from build123d import *

# Parameters (mm, degrees)
F0_R          = 3
F0_R_2        = 2.5
F1_DEPTH      = 408.599
F2_R          = 2
F3_R          = 7
F5_DEPTH      = 30
F5_DEPTH_BACK = 30


# Not quite as in the source:
# - a feature names something its author has since deleted; it is built from what else it names


with BuildPart() as f1:
    # F0 (on Top) → F1 (new body)
    with BuildSketch(Plane.XY):
        with BuildLine():
            Line((18.15, -30), (30, -30))
            Line((30, -30), (30, -18.15))
            Line((30, -18.15), (27.5, -18.15))
            Line((27.5, -18.15), (27.5, -20.15))
            Line((27.5, -20.15), (21.5477069044, -20.15))
            ThreePointArc((21.5477069044, -20.15), (19.5, -15), (21.5477069044, -9.85))
            Line((21.5477069044, -9.85), (27.5, -9.85))
            Line((27.5, -9.85), (27.5, -11.85))
            Line((27.5, -11.85), (30, -11.85))
            Line((30, -11.85), (30, 11.85))
            Line((30, 11.85), (27.5, 11.85))
            Line((27.5, 11.85), (27.5, 9.85))
            Line((27.5, 9.85), (21.5477069044, 9.85))
            ThreePointArc((21.5477069044, 9.85), (19.5, 15), (21.5477069044, 20.15))
            Line((21.5477069044, 20.15), (27.5, 20.15))
            Line((27.5, 20.15), (27.5, 18.15))
            Line((27.5, 18.15), (30, 18.15))
            Line((30, 18.15), (30, 30))
            Line((30, 30), (18.15, 30))
            Line((18.15, 30), (18.15, 27.5))
            Line((18.15, 27.5), (20.15, 27.5))
            Line((20.15, 27.5), (20.15, 21.5477069044))
            ThreePointArc((20.15, 21.5477069044), (15, 19.5), (9.85, 21.5477069044))
            Line((9.85, 21.5477069044), (9.85, 27.5))
            Line((9.85, 27.5), (11.85, 27.5))
            Line((11.85, 27.5), (11.85, 30))
            Line((11.85, 30), (-11.85, 30))
            Line((-11.85, 30), (-11.85, 27.5))
            Line((-11.85, 27.5), (-9.85, 27.5))
            Line((-9.85, 27.5), (-9.85, 21.5477069044))
            ThreePointArc((-9.85, 21.5477069044), (-15, 19.5), (-20.15, 21.5477069044))
            Line((-20.15, 21.5477069044), (-20.15, 27.5))
            Line((-20.15, 27.5), (-18.15, 27.5))
            Line((-18.15, 27.5), (-18.15, 30))
            Line((-18.15, 30), (-30, 30))
            Line((-30, 30), (-30, 18.15))
            Line((-30, 18.15), (-27.5, 18.15))
            Line((-27.5, 18.15), (-27.5, 20.15))
            Line((-27.5, 20.15), (-21.5477069044, 20.15))
            ThreePointArc((-21.5477069044, 20.15), (-19.5, 15), (-21.5477069044, 9.85))
            Line((-21.5477069044, 9.85), (-27.5, 9.85))
            Line((-27.5, 9.85), (-27.5, 11.85))
            Line((-27.5, 11.85), (-30, 11.85))
            Line((-30, 11.85), (-30, -11.85))
            Line((-30, -11.85), (-27.5, -11.85))
            Line((-27.5, -11.85), (-27.5, -9.85))
            Line((-27.5, -9.85), (-21.5477069044, -9.85))
            ThreePointArc((-21.5477069044, -9.85), (-19.5, -15), (-21.5477069044, -20.15))
            Line((-21.5477069044, -20.15), (-27.5, -20.15))
            Line((-27.5, -20.15), (-27.5, -18.15))
            Line((-27.5, -18.15), (-30, -18.15))
            Line((-30, -18.15), (-30, -30))
            Line((-30, -30), (-18.15, -30))
            Line((-18.15, -30), (-18.15, -27.5))
            Line((-18.15, -27.5), (-20.15, -27.5))
            Line((-20.15, -27.5), (-20.15, -21.5477069044))
            ThreePointArc((-20.15, -21.5477069044), (-15, -19.5), (-9.85, -21.5477069044))
            Line((-9.85, -21.5477069044), (-9.85, -27.5))
            Line((-9.85, -27.5), (-11.85, -27.5))
            Line((-11.85, -27.5), (-11.85, -30))
            Line((-11.85, -30), (11.85, -30))
            Line((11.85, -30), (11.85, -27.5))
            Line((11.85, -27.5), (9.85, -27.5))
            Line((9.85, -27.5), (9.85, -21.5477069044))
            ThreePointArc((9.85, -21.5477069044), (15, -19.5), (20.15, -21.5477069044))
            Line((20.15, -21.5477069044), (20.15, -27.5))
            Line((20.15, -27.5), (18.15, -27.5))
            Line((18.15, -27.5), (18.15, -30))
        make_face()
        with Locations((-25, -25)):
            Circle(F0_R, mode=Mode.SUBTRACT)
        with Locations((-15, -15)):
            Circle(F0_R_2, mode=Mode.SUBTRACT)
        with Locations((25, -25)):
            Circle(F0_R, mode=Mode.SUBTRACT)
        with Locations((15, -15)):
            Circle(F0_R_2, mode=Mode.SUBTRACT)
        with Locations((-25, 25)):
            Circle(F0_R, mode=Mode.SUBTRACT)
        with Locations((-15, 15)):
            Circle(F0_R_2, mode=Mode.SUBTRACT)
        Polygon((-7, 22), (-7, 27.5), (0, 27.5), (7, 27.5), (7, 22), (10, 16), (10, 10), (16, 10), (22, 7), (27.5, 7), (27.5, 0), (27.5, -7), (22, -7), (16, -10), (10, -10), (10, -16), (7, -22), (7, -27.5), (0, -27.5), (-7, -27.5), (-7, -22), (-10, -16), (-10, -10), (-16, -10), (-22, -7), (-27.5, -7), (-27.5, 0), (-27.5, 7), (-22, 7), (-16, 10), (-10, 10), (-10, 16), align=None, mode=Mode.SUBTRACT)
        with Locations((15, 15)):
            Circle(F0_R_2, mode=Mode.SUBTRACT)
        with Locations((25, 25)):
            Circle(F0_R, mode=Mode.SUBTRACT)
    extrude(amount=F1_DEPTH)

    # F2
    f2_edges = [f1.edges().sort_by_distance(p)[0] for p in [
        (-7, 27.5, 204.2995),
        (7, 27.5, 204.2995),
    ]]
    fillet(f2_edges, radius=F2_R)

    # F3
    f3_edges = [f1.edges().sort_by_distance(p)[0] for p in [
        (-10, 16, 204.2995),
        (10, 16, 204.2995),
    ]]
    fillet(f3_edges, radius=F3_R)

    # F4 (on Right) → F5 (cut, two sides)
    with BuildSketch(Plane.YZ) as f5_sk:
        Polygon((-164.2855995683, 38.6458085579), (-188.5911429791, -83.5464097089), (5.6944565892, -122.1922182668), (30, 0), align=None)
    extrude(amount=F5_DEPTH, mode=Mode.SUBTRACT)
    extrude(f5_sk.sketch, amount=-F5_DEPTH_BACK, mode=Mode.SUBTRACT)


solid = f1.part
Read the model definition and answer for the solid it produces. Units are mm, in the model's axes. A direction names the side the tool comes from. Give positions to 0.01 mm unless a question says otherwise; leave off trailing zeros. Write each loop counter-clockwise with the first axis right and the second up, starting at its lowest first coordinate (ties: lowest second). Pieces come first, ordered by that corner, then holes. Notation, with made-up numbers: (2, -27) -> (59, -27) arc R16 cw to (59, -14) -> close; hole circle Ø2 at (-39, 53). An arc over 180 degrees is marked (long way). Answer as a JSON object with one key per item and string values. Group by question number.
1) The mould has two halves that part along Y. Classify faces 3 (the flat face through (27.5, 0, 204)), 4 (the flat face through (0, 30, 201)), 5 (the flat face through (-10.97, -10.97, 8.15)): +Y half, -Y half, draft (parallel to the pull), parting line (faces both ways), or undercut.
2) Find section B-B (z = 297.5). Count the separate pieces of the cut face and the enclosed holes in it, and give its area (3 significant figures).
3) Consider L1, parallel to Y at x = -15, z = 207; L2, parallel to X at y = -25, z = 96. Determine where each line is inside the solid, lowest interval first. Write a range as from..to.
4) A tool of negligible diameter and unlimited length cuts with its end or side. For faces 1 (the flat face through (24, -30, 207)), 2 (the flat face through (0, 27.5, 202)), from which of +Z, -Z, +X, -X, +Y, -Y can it reach the whole face along a straight path? Write none if from no direction.
5) Find section A-A (y = -3). Write down the section's boundary in (x, z).
6) Each of these flat-tipped pins is pushed along its axis until it touches: P1, Ø3, axis at y = -14.5, z = 233.5, coming from the +X side; P2, Ø2, axis at x = 12, y = 14, coming from the -Z side; P3, Ø1.5, axis at x = -13, z = 167.5, coming from the +Y side. Where does it stop, or does it pass through?
Values follow:
{
 "1": {"face 3": "undercut", "face 4": "+Y half", "face 5": "-Y half"},
 "2": {"separate pieces": "1", "enclosed holes": "9", "area": "1,080 mm2"},
 "3": {"L1": "y = -19.5..-17.5, -12.5..-10, 10..12.5, 17.5..19.5", "L2": "x = -30..-28, -22..-20.15, -9.85..-7, 7..9.85, 20.15..22, 28..30"},
 "4": {"face 1": "+Z, -Z, +X, -X, -Y", "face 2": "+Z, -Z"},
 "5": {"outline": "(-30, 6.56) -> (-27.5, 6.56) -> (-27.5, 408.6) -> (-30, 408.6) -> close; (27.5, 6.56) -> (30, 6.56) -> (30, 408.6) -> (27.5, 408.6) -> close"},
 "6": {"P1": "stops at x = 19.77", "P2": "stops at z = 2.98", "P3": "stops at y = 20.02"}
}
